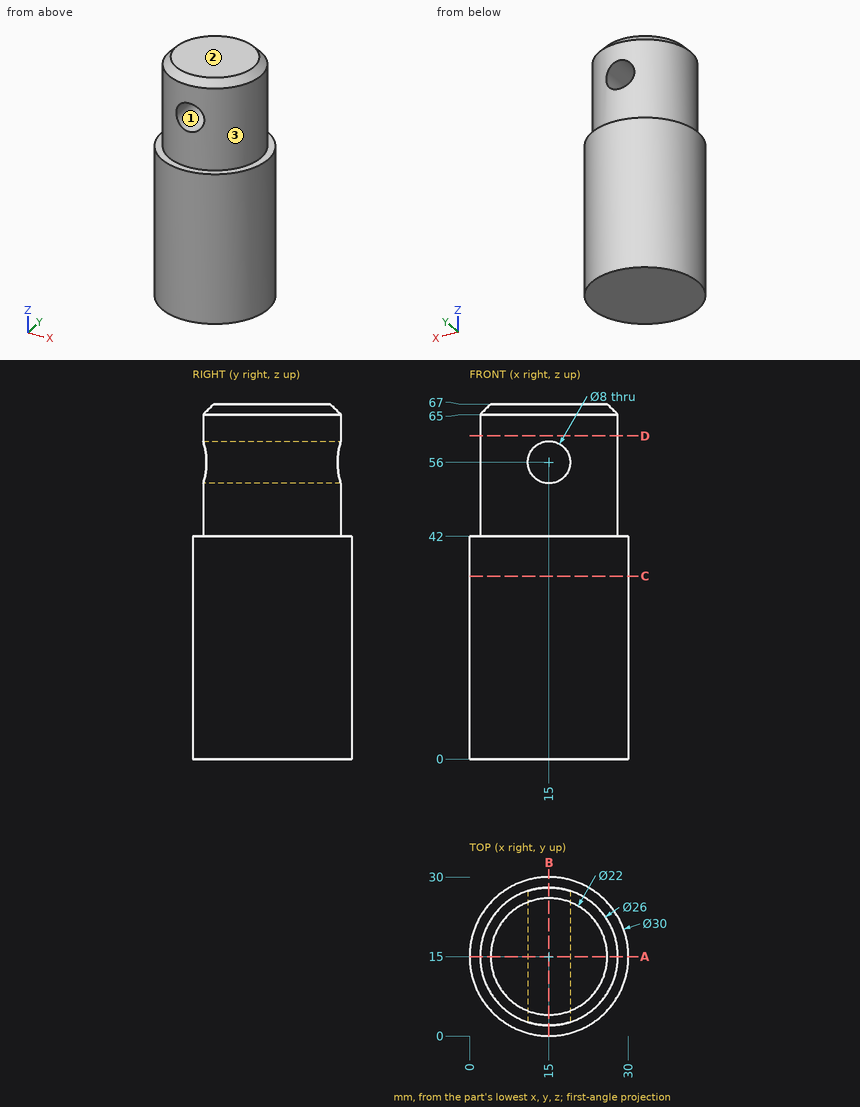
Drawing for the job (mm, zero at the part's lowest x, y, z). Coordinates: 2 decimals unless noted, no trailing zeros. Loops run counter-clockwise (first coordinate to the right, second up) from the corner with the lowest first, then second, coordinate; pieces in that order, holes last. Notation, with made-up numbers: (-32, -19.5) - (-17, -19.5) arc R26 cw to (-17, 16.5) - close; hole circle Ø2 at (8.5, -30). An arc over 180 degrees is marked (long way). Return JSON: item names as keys, results as strings.
1. Mould opens along X. For the marked faces 1, 2 and 3 say: released by +X, released by -X, zero draft, split by the parting line, or undercut.
Result:
{"face 1": "undercut", "face 2": "zero draft", "face 3": "split by the parting line"}
2. Band-saw the part on C-C (z = 34.5). Give the cut face in (x, y), and give its area (3 significant figures).
Result:
{"outline": "circle Ø30 at (15, 15)", "area": "707 mm2"}
3. Drop flat-ended pins along their axis: pin 1 (10 mm diameter, centred on y = 7, z = 34, fed in from -X); pin 2 (10.5 mm diameter, centred on x = 15, z = 56, fed in from +Y); pin 3 (4 mm diameter, centred on x = 20.5, z = 57, fed in from +Y). Give the stop position or say it passes through.
Result:
{"pin 1": "stops at x = 0.3", "pin 2": "stops at y = 28", "pin 3": "stops at y = 27.48"}
4. Band-saw the part on B-B (x = 15). Give the cut face in (y, z), and give its area (3 significant figures).
Result:
{"outline": "(0, 0) - (30, 0) - (30, 42) - (28, 42) - (28, 52) - (2, 52) - (2, 42) - (0, 42) - close; (2, 60) - (28, 60) - (28, 65) - (26, 67) - (4, 67) - (2, 65) - close", "area": "1,700 mm2"}
5. Probe L1, parallel to Z at x = 15, y = 17.5; L2, parallel to Z at x = 13, y = 23.25; L3, parallel to X at y = 11.75, z = 56. List the from-to ranges inside material, lowest first. Write a range as from..to.
Result:
{"L1": "z = 0..52, 60..67", "L2": "z = 0..52.54, 59.46..67", "L3": "x = 2.41..11, 19..27.59"}
6. Band-saw the part on A-A (y = 15). Give the cut face in (x, z).
Result:
{"outline": "(0, 0) - (30, 0) - (30, 42) - (28, 42) - (28, 65) - (26, 67) - (4, 67) - (2, 65) - (2, 42) - (0, 42) - close; hole circle Ø8 at (15, 56)"}
7. Band-saw the part on D-D (z = 61). Give the cut face in (x, y).
Result:
{"outline": "circle Ø26 at (15, 15)"}
